```python
from build123d import *
from build123d.topology import SkipClean

# Parameters (mm, degrees)
BOSS_EXTRUDE1_DEPTH   = 11
BOSS_EXTRUDE1_2_DEPTH = 11
BOSS_EXTRUDE1_3_DEPTH = 11
BOSS_EXTRUDE1_4_DEPTH = 11
BOSS_EXTRUDE1_5_DEPTH = 11
BOSS_EXTRUDE1_6_DEPTH = 11
SKETCH1_R             = 15
BOSS_EXTRUDE1_7_DEPTH = 11
BOSS_EXTRUDE1_8_DEPTH = 11
SKETCH1_3_R           = 15
SKETCH1_3_R_2         = 20
SKETCH1_3_R_3         = 40
SKETCH1_3_R_4         = 16
BOSS_EXTRUDE2_DEPTH   = 25


with BuildPart() as part:
    # Sketch1 → Boss-Extrude1 (new body)
    with BuildSketch(Plane.XY):
        with BuildLine():
            ThreePointArc((13.379398651, 16.186157411), (18.186533479, 10.5), (20.707322833, 3.493820414))
            Line((20.707322833, 3.493820414), (31.808697221, 3.493820414))
            ThreePointArc((31.808697221, 3.493820414), (27.712812921, 16), (18.930085845, 25.800229648))
            Line((18.930085845, 25.800229648), (13.379398651, 16.186157411))
        make_face()
    extrude(amount=BOSS_EXTRUDE1_DEPTH)



with BuildPart() as body_2:
    # Sketch1 → Boss-Extrude1 2 (new body)
    with BuildSketch(Plane.XY):
        with BuildLine():
            Line((31.808697221, -3.493820414), (20.707322833, -3.493820414))
            ThreePointArc((20.707322833, -3.493820414), (18.186533479, -10.5), (13.379398651, -16.186157411))
            Line((13.379398651, -16.186157411), (18.930085845, -25.800229648))
            ThreePointArc((18.930085845, -25.800229648), (27.712812921, -16), (31.808697221, -3.493820414))
        make_face()
    extrude(amount=BOSS_EXTRUDE1_2_DEPTH)


with BuildPart() as body_3:
    # Sketch1 → Boss-Extrude1 3 (new body)
    with BuildSketch(Plane.XY):
        with BuildLine():
            Line((12.878611376, -29.294050062), (7.327924182, -19.679977825))
            ThreePointArc((7.327924182, -19.679977825), (0, -21), (-7.327924182, -19.679977825))
            Line((-7.327924182, -19.679977825), (-12.878611376, -29.294050062))
            ThreePointArc((-12.878611376, -29.294050062), (0, -32), (12.878611376, -29.294050062))
        make_face()
    extrude(amount=BOSS_EXTRUDE1_3_DEPTH)


with BuildPart() as body_4:
    # Sketch1 → Boss-Extrude1 4 (new body)
    with BuildSketch(Plane.XY):
        with BuildLine():
            Line((-18.930085845, -25.800229648), (-13.379398651, -16.186157411))
            ThreePointArc((-13.379398651, -16.186157411), (-18.186533479, -10.5), (-20.707322833, -3.493820414))
            Line((-20.707322833, -3.493820414), (-31.808697221, -3.493820414))
            ThreePointArc((-31.808697221, -3.493820414), (-27.712812921, -16), (-18.930085845, -25.800229648))
        make_face()
    extrude(amount=BOSS_EXTRUDE1_4_DEPTH)


with BuildPart() as body_5:
    # Sketch1 → Boss-Extrude1 5 (new body)
    with BuildSketch(Plane.XY):
        with BuildLine():
            Line((-31.808697221, 3.493820414), (-20.707322833, 3.493820414))
            ThreePointArc((-20.707322833, 3.493820414), (-18.186533479, 10.5), (-13.379398651, 16.186157411))
            Line((-13.379398651, 16.186157411), (-18.930085845, 25.800229648))
            ThreePointArc((-18.930085845, 25.800229648), (-27.712812921, 16), (-31.808697221, 3.493820414))
        make_face()
    extrude(amount=BOSS_EXTRUDE1_5_DEPTH)


with BuildPart() as body_6:
    # Sketch1 → Boss-Extrude1 6 (new body)
    with BuildSketch(Plane.XY):
        with BuildLine():
            Line((-12.878611376, 29.294050062), (-7.327924182, 19.679977825))
            ThreePointArc((-7.327924182, 19.679977825), (0, 21), (7.327924182, 19.679977825))
            Line((7.327924182, 19.679977825), (12.878611376, 29.294050062))
            ThreePointArc((12.878611376, 29.294050062), (0, 32), (-12.878611376, 29.294050062))
        make_face()
    extrude(amount=BOSS_EXTRUDE1_6_DEPTH)


with BuildPart() as body_7:
    # Sketch1 → Boss-Extrude1 7 (new body)
    with BuildSketch(Plane.XY):
        with BuildLine():
            Line((106.793251867, 10.862167911), (67.63291446, 71.405276307))
            ThreePointArc((67.63291446, 71.405276307), (43.887296944, 80.090666025), (29.002885891, 59.651863383))
            ThreePointArc((29.002885891, 59.651863383), (22.168588856, 44.262528341), (6.003756239, 39.546869801))
            ThreePointArc((6.003756239, 39.546869801), (39.99999995, 0.002005859), (6.007722482, -39.546267467))
            ThreePointArc((6.007722482, -39.546267467), (22.304723723, -44.376428641), (29, -60))
            ThreePointArc((29, -60), (44.054043545, -80.140645517), (67.63291446, -71.405276307))
            Line((67.63291446, -71.405276307), (106.793251867, -10.862167911))
            ThreePointArc((106.793251867, -10.862167911), (70, 0), (106.793251867, 10.862167911))
        make_face()
        with Locations((50, -60)):
            Circle(SKETCH1_R, mode=Mode.SUBTRACT)
        with Locations((50, 60)):
            Circle(SKETCH1_R, mode=Mode.SUBTRACT)
    extrude(amount=BOSS_EXTRUDE1_7_DEPTH)


with BuildPart() as body_8:
    # Sketch1 → Boss-Extrude1 8 (new body)
    with BuildSketch(Plane.XY):
        with BuildLine():
            ThreePointArc((-6.007722482, -39.546267467), (-39.99999995, 0.002005859), (-6.003756239, 39.546869801))
            ThreePointArc((-6.003756239, 39.546869801), (-22.168588856, 44.262528341), (-29.002885891, 59.651863383))
            ThreePointArc((-29.002885891, 59.651863383), (-43.887296944, 80.090666025), (-67.63291446, 71.405276307))
            Line((-67.63291446, 71.405276307), (-106.793251867, 10.862167911))
            ThreePointArc((-106.793251867, 10.862167911), (-110, 0), (-106.793251867, -10.862167911))
            Line((-106.793251867, -10.862167911), (-67.63291446, -71.405276307))
            ThreePointArc((-67.63291446, -71.405276307), (-44.054043545, -80.140645517), (-29, -60))
            ThreePointArc((-29, -60), (-22.304723723, -44.376428641), (-6.007722482, -39.546267467))
        make_face()
        with Locations((-50, -60)):
            Circle(SKETCH1_R, mode=Mode.SUBTRACT)
    extrude(amount=BOSS_EXTRUDE1_8_DEPTH)


with BuildPart() as part_1:
    with SkipClean():  # the faces are left unmerged after this step: merging them gives an invalid solid
        add(part.part)

        add(body_2.part)  # Boss-Extrude2 merges body 2

        add(body_3.part)  # Boss-Extrude2 merges body 3

        add(body_4.part)  # Boss-Extrude2 merges body 4

        add(body_5.part)  # Boss-Extrude2 merges body 5

        add(body_6.part)  # Boss-Extrude2 merges body 6

        add(body_7.part)  # Boss-Extrude2 merges body 7

        add(body_8.part)  # Boss-Extrude2 merges body 8
        # Sketch1_3 → Boss-Extrude2 (add, symmetric)
        # profile 1 of 7: a face of its own
        with BuildSketch(Plane.XY):
            with Locations((50, 60)):
                Circle(SKETCH1_3_R)
        # profile 2 of 7: a face of its own
        with BuildSketch(Plane.XY):
            with Locations((50, -60)):
                Circle(SKETCH1_3_R)
        # profile 3 of 7: a face of its own
        with BuildSketch(Plane.XY):
            with Locations((-50, -60)):
                Circle(SKETCH1_3_R)
        # profile 4 of 7: a face of its own
        with BuildSketch(Plane.XY):
            with Locations((-90, 0)):
                Circle(SKETCH1_3_R_2)
            with Locations((-90, 0)):
                Circle(SKETCH1_3_R, mode=Mode.SUBTRACT)
        # profile 5 of 7: a face of its own
        with BuildSketch(Plane.XY):
            Circle(SKETCH1_3_R_3)
            Circle(SKETCH1_3_R_4, mode=Mode.SUBTRACT)
            with BuildLine():
                ThreePointArc((-12.878611376, -29.294050062), (0, -32), (12.878611376, -29.294050062))
                Line((12.878611376, -29.294050062), (7.327924182, -19.679977825))
                ThreePointArc((7.327924182, -19.679977825), (0, -21), (-7.327924182, -19.679977825))
                Line((-7.327924182, -19.679977825), (-12.878611376, -29.294050062))
            make_face(mode=Mode.SUBTRACT)
            with BuildLine():
                ThreePointArc((18.930085845, -25.800229648), (27.712812921, -16), (31.808697221, -3.493820414))
                Line((31.808697221, -3.493820414), (20.707322833, -3.493820414))
                ThreePointArc((20.707322833, -3.493820414), (18.186533479, -10.5), (13.379398651, -16.186157411))
                Line((13.379398651, -16.186157411), (18.930085845, -25.800229648))
            make_face(mode=Mode.SUBTRACT)
            with BuildLine():
                ThreePointArc((12.878611376, 29.294050062), (0, 32), (-12.878611376, 29.294050062))
                Line((-12.878611376, 29.294050062), (-7.327924182, 19.679977825))
                ThreePointArc((-7.327924182, 19.679977825), (0, 21), (7.327924182, 19.679977825))
                Line((7.327924182, 19.679977825), (12.878611376, 29.294050062))
            make_face(mode=Mode.SUBTRACT)
            with BuildLine():
                ThreePointArc((31.808697221, 3.493820414), (27.712812921, 16), (18.930085845, 25.800229648))
                Line((18.930085845, 25.800229648), (13.379398651, 16.186157411))
                ThreePointArc((13.379398651, 16.186157411), (18.186533479, 10.5), (20.707322833, 3.493820414))
                Line((20.707322833, 3.493820414), (31.808697221, 3.493820414))
            make_face(mode=Mode.SUBTRACT)
            with BuildLine():
                Line((-13.379398651, 16.186157411), (-18.930085845, 25.800229648))
                ThreePointArc((-18.930085845, 25.800229648), (-27.712812921, 16), (-31.808697221, 3.493820414))
                Line((-31.808697221, 3.493820414), (-20.707322833, 3.493820414))
                ThreePointArc((-20.707322833, 3.493820414), (-18.186533479, 10.5), (-13.379398651, 16.186157411))
            make_face(mode=Mode.SUBTRACT)
            with BuildLine():
                Line((-20.707322833, -3.493820414), (-31.808697221, -3.493820414))
                ThreePointArc((-31.808697221, -3.493820414), (-27.712812921, -16), (-18.930085845, -25.800229648))
                Line((-18.930085845, -25.800229648), (-13.379398651, -16.186157411))
                ThreePointArc((-13.379398651, -16.186157411), (-18.186533479, -10.5), (-20.707322833, -3.493820414))
            make_face(mode=Mode.SUBTRACT)
        # profile 6 of 7: a face of its own
        with BuildSketch(Plane.XY):
            with Locations((90, 0)):
                Circle(SKETCH1_3_R_2)
        # profile 7 of 7: a face of its own
        with BuildSketch(Plane.XY):
            with Locations(Location((-50, 60, 0), (0, 0, 180))):
                Circle(SKETCH1_3_R)
        extrude(amount=BOSS_EXTRUDE2_DEPTH, both=True)


solid = part_1.part
```
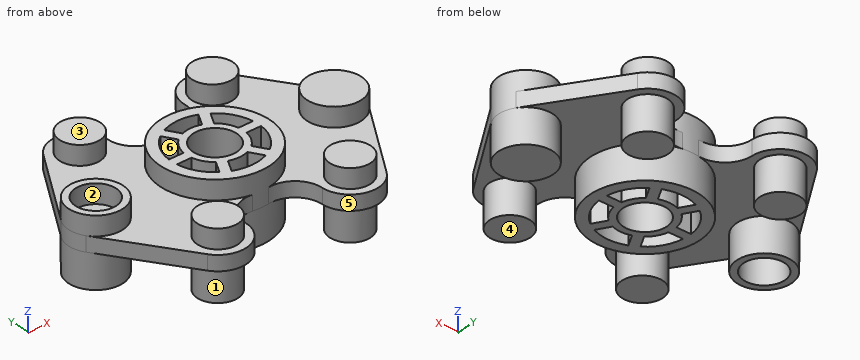
Build history of the part. All positions in model axes, mm. Face numbers are marked on the shaded views. A direction names the side the tool comes from. Round coordinates to 2 decimals unless told otherwise and drop trailing zeros. Write each loop counter-clockwise with the first axis right and the second up, starting at its lowest first coordinate (ties: lowest second). Pieces come first, ordered by that corner, then holes.
1) Band-saw the part on C-C, the plane x = 0. List the corners of the cut face in (y, z), and give its area (3 significant figures).
2) Band-saw the part on A-A, the plane z = 14. Give the number of separate pieces and of enclosed holes in the cut face, and give its area (3 significant figures).
3) Pin check, flat tips, straight feed: pin 1 (8 mm diameter, centred on x = 84, z = -19, fed in from +Y); pin 2 (8 mm diameter, centred on x = -81.5, z = -15.5, fed in from +Y); pin 3 (9 mm diameter, centred on x = -27.5, z = 16, fed in from +Y). Stop position of each tip, or through.
4) 3-axis set-ups, long thin cutter, end or side, ignore diameter. For the marked faces 1, 2 and 3: which of +Z, -Z, +X, -X, +Y, -Y reach the whole face in a straight line?
5) Band-saw the part on D-D, the plane x = -95. List the corners of the cut face in (y, z).
6) Mould opens along Y. For the marked faces 4, 5 and 6 say: +Y half, -Y half, draft (parallel to the pull), parting line (faces both ways), or undercut.
7) Drill centre lines: probe 1 along X at (y, z) = (16.5, -14); probe 2 along Y at (x, z) = (23, -8.5); probe 3 along Y at (x, z) = (-90, 15). Where is each one in solid material? Low to high.
Ans:
1. outline: (-40, -25) - (-32, -25) - (-32, 0) - (-21, 0) - (-21, -25) - (-16, -25) - (-16, 25) - (-21, 25) - (-21, 11) - (-32, 11) - (-32, 25) - (-40, 25) - close; (16, -25) - (21, -25) - (21, 0) - (32, 0) - (32, -25) - (40, -25) - (40, 25) - (32, 25) - (32, 11) - (21, 11) - (21, 25) - (16, 25) - close
1. area: 1,540 mm2
2. separate pieces: 7
2. enclosed holes: 8
2. area: 7,490 mm2
3. pin 1: stops at y = 19.9
3. pin 2: stops at y = 19.49
3. pin 3: stops at y = 32.73
4. face 1: -Z
4. face 2: +Z
4. face 3: +Z, +X, -X, +Y, -Y
5. outline: (-29.09, 0) - (-19.36, 0) - (-19.36, -25) - (-14.14, -25) - (-14.14, 0) - (14.14, 0) - (14.14, -25) - (19.36, -25) - (19.36, 0) - (29.09, 0) - (29.09, 11) - (19.36, 11) - (19.36, 25) - (14.14, 25) - (14.14, 11) - (-14.14, 11) - (-14.14, 25) - (-19.36, 25) - (-19.36, 11) - (-29.09, 11) - close
6. face 4: draft
6. face 5: -Y half
6. face 6: undercut
7. probe 1: x = -101.3 to -78.7, -36.44 to -27.42, -13.56 to 13.56, 27.42 to 36.44, 78.7 to 101.3
7. probe 2: y = -32.73 to -22.25, -3.49 to 3.49, 22.25 to 32.73
7. probe 3: y = -20 to -15, 15 to 20
